Design review of the part built by this model. Coordinates are the model's own, in mm. Give positions to 0.01 mm unless a question says otherwise; leave off trailing zeros. Write each loop counter-clockwise with the first axis right and the second up, starting at its lowest first coordinate (ties: lowest second). Pieces come first, ordered by that corner, then holes. Notation, with made-up numbers: (12.25, 44) -> (55.25, 44) arc R26 ccw to (55.25, 71) -> close; hole circle Ø5 at (8, 40). An arc over 180 degrees is marked (long way). Write each question's results on one line, items separated by ' | '. Start each with the question number.
(1) Clearance check with flat-ended pins moving along their axes: pin 1 (3 mm diameter, centred on x = -3, y = 2, fed in from -Z); pin 2 (2.5 mm diameter, centred on y = 0, z = 23, fed in from +X); pin 3 (3 mm diameter, centred on x = -8, y = 1, fed in from +Z); pin 4 (1.5 mm diameter, centred on x = -1, y = -2.5, fed in from +Z). State where each tip first meets the part, or that it passes through.
(2) Take a section at B-B (z = 23). State the section outline as (x, y) points.
(3) To check wall thickness, follow probe 1 along Y at (x, z) = (19, 23.25); probe 2 along Z at (x, y) = (17, -0.5); probe 3 along Y at (x, z) = (11.5, 23). State the ranges of each line that lie inside material, in increasing order.
(4) Take a section at A-A (y = 0). State the section outline as (x, z) points.
(5) Take a section at D-D (x = -18). State the section outline as (y, z) points, plus the area to 3 significant figures.
(6) Take a section at C-C (x = 20.5). State the section outline as (y, z) points, plus the area to 3 significant figures.
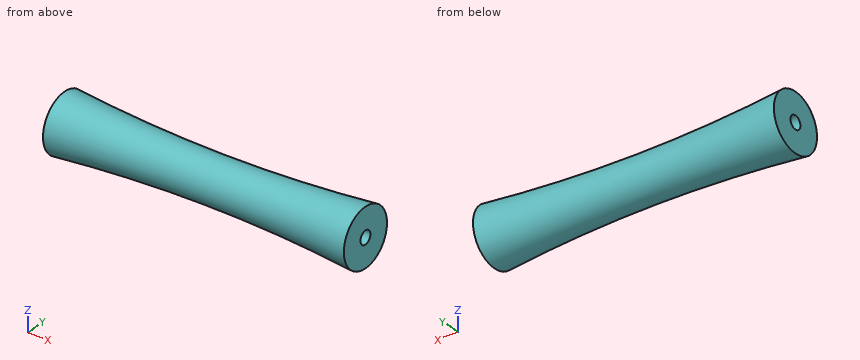
Autodesk Inventor part; units mm, degrees
ref_plane "YZ Plane" through (0, 0, 0) normal (1, 0, 0) x (0, 1, 0)
ref_plane "XZ Plane" through (0, 0, 0) normal (0, 1, 0) x (-1, 0, 0)
ref_plane "XY Plane" through (0, 0, 0) normal (0, 0, 1) x (1, 0, 0)
sketch "Sketch1" plane through (0, 0, 0) normal (0, 1, 0) x (-1, 0, 0)
  line L0 (24, 18.5) -> (24, 23)
  line L1 (24, 23) -> (-24, 23)
  line L2 (-24, 23) -> (-24, 18.5)
  arc A0 (24, 18.5) -> (-24, 18.5) centre (0, -220.297) ccw
  point P0 (0, 0)
  dimension "d9" = 4.5
  dimension "d10" = 240
revolve "Revolution1" add sketch "Sketch1" angle 360 about axis through (-24, 0, 23) along (1, 0, 0)
sketch "Sketch2" plane through (24, 0, 23) normal (1, 0, 0) x (0, 0, -1)
  circle A0 centre (0, 0) radius 4.5
  circle A1 centre (0, 0) radius 1.01
  point P0 (23, 0)
  dimension "d12" = 2.02
extrude "Extrusion1" cut sketch "Sketch2" against normal blind 48 contours A1
sketch "Sketch4" plane through (-24, 0, 23) normal (-1, 0, 0) x (0, 0, 1)
  circle A0 centre (0, 0) radius 1.01
  circle A1 centre (0, 0) radius 4.5
  point P0 (-23, 0)
extrude "Extrusion2" cut sketch "Sketch4" against normal blind 1
sketch "Sketch5" plane through (24, 0, 23) normal (1, 0, 0) x (0, 0, -1)
  circle A0 centre (0, 0) radius 1.01
  circle A1 centre (0, 0) radius 4.5
  point P0 (23, 0)
extrude "Extrusion3" cut sketch "Sketch5" against normal blind 1 contours A0 | A1
properties part number "Roller"
Report:
1) pin 1: z = 19.72 | pin 2: x = 23 | pin 3: z = 26.47 | pin 4: z = 25.8
2) outline: (-23, -4.4) arc R240 cw to (23, -4.4) -> (23, -1.01) -> (-23, -1.01) -> close; (-23, 1.01) -> (23, 1.01) -> (23, 4.4) arc R240 cw to (-23, 4.4) -> close
3) probe 1: -4.04 to -0.98, 0.98 to 4.04 | probe 2: 19.13 to 22.12, 23.88 to 26.87 | probe 3: -3.57 to -1.01, 1.01 to 3.57
4) outline: (-23, 18.6) arc R240 cw to (23, 18.6) -> (23, 21.99) -> (-23, 21.99) -> close; (-23, 24.01) -> (23, 24.01) -> (23, 27.4) arc R240 cw to (-23, 27.4) -> close
5) outline: circle Ø7.95 at (0, 23); hole circle Ø2.02 at (0, 23) | area: 46.4 mm2
6) outline: circle Ø8.35 at (0, 23); hole circle Ø2.02 at (0, 23) | area: 51.5 mm2
